```python
from build123d import *

# Parameters (mm, degrees)
BOSS_EXTRUDE1_DEPTH      = 16
SKETCH2_R                = 15
SKETCH2_R_2              = 11
BOSS_EXTRUDE2_DEPTH      = 30
BOSS_EXTRUDE2_DEPTH_BACK = 35
SKETCH3_R                = 6.75
CUT_EXTRUDE1_DEPTH       = 8.75
SKETCH4_R                = 11
CUT_EXTRUDE2_DEPTH       = 24


with BuildPart() as part:
    # Sketch1 → Boss-Extrude1 (new body, symmetric)
    with BuildSketch(Plane.XY):
        with BuildLine():
            Line((-7, -15), (7, -15))
            ThreePointArc((7, -15), (14.071067812, -12.071067812), (17, -5))
            Line((17, -5), (17, 5))
            ThreePointArc((17, 5), (14.071067812, 12.071067812), (7, 15))
            Line((7, 15), (-7, 15))
            ThreePointArc((-7, 15), (-14.071067812, 12.071067812), (-17, 5))
            Line((-17, 5), (-17, -5))
            ThreePointArc((-17, -5), (-14.071067812, -12.071067812), (-7, -15))
        make_face()
    extrude(amount=BOSS_EXTRUDE1_DEPTH, both=True)

    # Sketch2 → Boss-Extrude2 (add, two sides)
    with BuildSketch(Plane(origin=(0, 0, 0), x_dir=(1, 0, 0), z_dir=(0, 1, 0))) as boss_extrude2_sk:
        Circle(SKETCH2_R)
        Circle(SKETCH2_R_2, mode=Mode.SUBTRACT)
    extrude(amount=BOSS_EXTRUDE2_DEPTH)
    extrude(boss_extrude2_sk.sketch, amount=-BOSS_EXTRUDE2_DEPTH_BACK)

    # Sketch3 → Cut-Extrude1 (cut)
    with BuildSketch(Plane(origin=(0, 0, -16), x_dir=(-1, 0, 0), z_dir=(0, 0, -1))):
        Circle(SKETCH3_R)
    cut_extrude1 = extrude(amount=-CUT_EXTRUDE1_DEPTH, mode=Mode.SUBTRACT)

    # Mirror1: Cut-Extrude1 across plane
    add(cut_extrude1.mirror(Plane.XY), mode=Mode.SUBTRACT)

    # Sketch4 → Cut-Extrude2 (cut)
    with BuildSketch(Plane(origin=(0, 30, 0), x_dir=(1, 0, 0), z_dir=(0, 1, 0))):
        Circle(SKETCH4_R)
    extrude(amount=-CUT_EXTRUDE2_DEPTH, mode=Mode.SUBTRACT)


solid = part.part
```
Read the model definition and answer for the solid it produces. Units are mm, in the model's axes. A direction names the side the tool comes from. Give positions to 0.01 mm unless a question says otherwise; leave off trailing zeros. Write each loop counter-clockwise with the first axis right and the second up, starting at its lowest first coordinate (ties: lowest second). Pieces come first, ordered by that corner, then holes. Notation, with made-up numbers: (75, -1) -> (123, -1) arc R11 ccw to (123, 8) -> close; hole circle Ø11 at (-21.5, 15.25). An arc over 180 degrees is marked (long way). Answer in a Markdown table with one row per item.
1) Section B-B on z = 0 is taken. Give the vertices of the cut face in (x, y), plus the area to 3 significant figures.
Results list:
| item | result |
|---|---|
| outline | (-17, -5) arc R10 ccw to (-15, -11) -> (-15, -35) -> (-11, -35) -> (-11, -14.17) arc R10 ccw to (-7, -15) -> (7, -15) arc R10 ccw to (11, -14.17) -> (11, -35) -> (15, -35) -> (15, -11) arc R10 ccw to (17, -5) -> (17, 5) arc R10 ccw to (15, 11) -> (15, 30) -> (11, 30) -> (11, 6) -> (-11, 6) -> (-11, 30) -> (-15, 30) -> (-15, 11) arc R10 ccw to (-17, 5) -> close |
| area | 1,050 mm^2 |
2) A tool of negligible diameter and unlimited length cuts with its end or side. For faces 4 (the cylindrical face through (15.128, -10.825, 0.224)), 5 (the cylindrical face through (15.25, 10.65, 0.22)), 6 (the cylindrical face through (-3.252, 22.478, 14.643)), from which of +Z, -Z, +X, -X, +Y, -Y can it reach the whole face along a straight path? Write none if from no direction.
Results list:
| item | result |
|---|---|
| face 4 | +X, -Y |
| face 5 | +X, +Y |
| face 6 | +Y |
3) Section A-A on x = 0 is taken. Give the vertices of the cut face in (y, z), plus the area to 3 significant figures.
Results list:
| item | result |
|---|---|
| outline | (-35, -15) -> (-15, -15) -> (-15, -16) -> (-6.75, -16) -> (-6.75, -7.25) -> (6, -7.25) -> (6, 7.25) -> (-6.75, 7.25) -> (-6.75, 16) -> (-15, 16) -> (-15, 15) -> (-35, 15) -> (-35, 11) -> (-15, 11) -> (-15, -11) -> (-35, -11) -> close; (6.75, -16) -> (15, -16) -> (15, -15) -> (30, -15) -> (30, -11) -> (6.75, -11) -> close; (6.75, 11) -> (30, 11) -> (30, 15) -> (15, 15) -> (15, 16) -> (6.75, 16) -> close |
| area | 811 mm^2 |
4) Straight lines are drawn through the part: line 1 (X direction, y = -25.5, z = 0); line 2 (X direction, y = 0, z = -11.25); line 3 (Y direction, x = 0, z = 13). For each, find the intervals that lie inside material, in ascending order. Write a range as [from, to].
Results list:
| item | result |
|---|---|
| line 1 | [-15, -11], [11, 15] |
| line 2 | [-17, -6.75], [6.75, 17] |
| line 3 | [-35, -6.75], [6.75, 30] |
5) Determine the mould class of faces 1 (the cylindrical face through (-2.38, -24.44, 10.74)), 2 (the flat face through (0.1, 15, -15.2)), 3 (the cylindrical face through (-11.056, -25.499, -10.138)) for opening direction Z: released by +Z, released by -Z, zero draft, split by the parting line, or undercut.
Results list:
| item | result |
|---|---|
| face 1 | undercut |
| face 2 | zero draft |
| face 3 | split by the parting line |
6) Each of these flat-tipped pins is pushed along its axis until it touches: pin 1 Ø5 at (y, z) = (11, 4) entering from +X; pin 2 Ø11 at (x, y) = (0, 0) entering from +Z; pin 3 Ø12 at (y, z) = (20, -7) entering from -X. Where does it stop, or does it pass through?
Results list:
| item | result |
|---|---|
| pin 1 | x = 16.37 |
| pin 2 | z = 7.25 |
| pin 3 | x = -14.97 |
7) Section C-C on y = 0 is taken. Give the vertices of the cut face in (x, z).
Results list:
| item | result |
|---|---|
| outline | (-17, -16) -> (-6.75, -16) -> (-6.75, -7.25) -> (6.75, -7.25) -> (6.75, -16) -> (17, -16) -> (17, 16) -> (6.75, 16) -> (6.75, 7.25) -> (-6.75, 7.25) -> (-6.75, 16) -> (-17, 16) -> close |
8) Section D-D on x = 4 is taken. Give the vertices of the cut face in (y, z), plus the area to 3 significant figures.
Results list:
| item | result |
|---|---|
| outline | (-35, -14.46) -> (-15, -14.46) -> (-15, -16) -> (-5.44, -16) -> (-5.44, -7.25) -> (5.44, -7.25) -> (5.44, -16) -> (15, -16) -> (15, -14.46) -> (30, -14.46) -> (30, -10.25) -> (6, -10.25) -> (6, 10.25) -> (30, 10.25) -> (30, 14.46) -> (15, 14.46) -> (15, 16) -> (5.44, 16) -> (5.44, 7.25) -> (-5.44, 7.25) -> (-5.44, 16) -> (-15, 16) -> (-15, 14.46) -> (-35, 14.46) -> (-35, 10.25) -> (-15, 10.25) -> (-15, -10.25) -> (-35, -10.25) -> close |
| area | 880 mm^2 |
